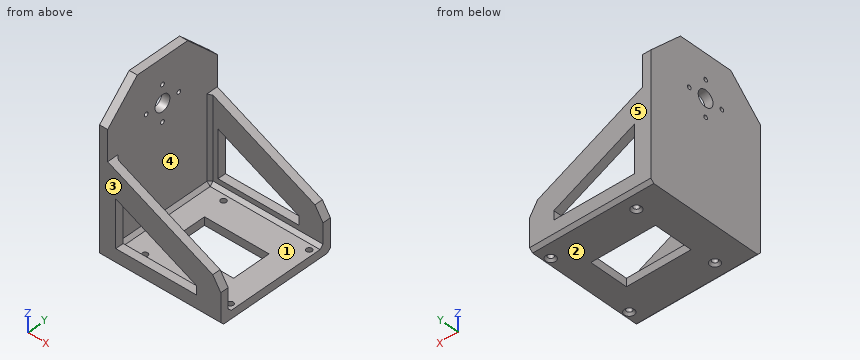
```python
from build123d import *

# Parameters (mm, degrees)
SKETCH004_W      = 75
SKETCH004_H      = 74
SKETCH004_W_2    = 40
SKETCH004_H_2    = 24
PAD_DEPTH        = 5
SKETCH006_W      = 74
SKETCH006_H      = 97
PAD003_DEPTH     = 5
PAD004_DEPTH     = 5
HOLE_D           = 3.4
HOLE_CSINK_D     = 6.1
HOLE_CSINK_ANGLE = 90
SKETCH002_R      = 5
SKETCH002_R_2    = 1.25
POCKET_DEPTH     = 5.001
CHAMFER_SIZE     = 2
CHAMFER001_SIZE  = 5.5
CHAMFER002_SIZE  = 20


with BuildPart() as part:
    # Sketch004 → Pad (new body)
    with BuildSketch(Plane.XY):
        with Locations((32.5, 0)):
            Rectangle(SKETCH004_W, SKETCH004_H)
        with Locations((35, 0)):
            Rectangle(SKETCH004_W_2, SKETCH004_H_2, mode=Mode.SUBTRACT)
    extrude(amount=-PAD_DEPTH)

    # Sketch006 → Pad003 (join)
    with BuildSketch(Plane.YZ):
        with Locations((0, 43.5)):
            Rectangle(SKETCH006_W, SKETCH006_H)
    extrude(amount=-PAD003_DEPTH)

    # Sketch001 → Pad004 (join)
    with BuildSketch(Plane.XZ.offset(37)):
        Polygon((-5, 55.5), (70, 20), (70, -5), (-5, -5), align=None)
        Polygon((5, 34.171185), (55, 10.504519), (55, 5), (5, 5), align=None, mode=Mode.SUBTRACT)
    pad004 = extrude(amount=-PAD004_DEPTH)

    # Mirrored: Pad004 across XZ
    add(pad004.mirror(Plane.XZ))

    # Hole (through all)
    with Locations(Plane(origin=(0, 0, -5), x_dir=(1, 0, 0), z_dir=(0, 0, -1))):
        with Locations((66.5, -26.5), (13.5, -26.5), (13.5, 26.5), (66.5, 26.5)):
            CounterSinkHole(HOLE_D / 2, HOLE_CSINK_D / 2, counter_sink_angle=HOLE_CSINK_ANGLE)

    # Sketch002 → Pocket (cut, through all)
    with BuildSketch(Plane.YZ):
        with Locations((0, 65.5)):
            Circle(SKETCH002_R)
        with Locations((0, 76.5)):
            Circle(SKETCH002_R_2)
        with Locations((11, 65.5)):
            Circle(SKETCH002_R_2)
        with Locations((0, 54.5)):
            Circle(SKETCH002_R_2)
        with Locations((-11, 65.5)):
            Circle(SKETCH002_R_2)
    extrude(amount=-POCKET_DEPTH, mode=Mode.SUBTRACT)

    # Chamfer
    chamfer_edges = [part.edges().sort_by_distance(p)[0] for p in [
        (0, 0, 0),
        (35, 32, 0),
        (35, -32, 0),
        (0, -32, 26.566667),
        (0, 32, 26.566667),
        (32.5, -37, -5),
        (32.5, 37, -5),
    ]]
    chamfer(chamfer_edges, length=CHAMFER_SIZE)

    # Chamfer001
    chamfer001_edges = [part.edges().sort_by_distance(p)[0] for p in [
        (70, -34.5, 20),
        (70, 34.5, 20),
    ]]
    chamfer(chamfer001_edges, length=CHAMFER001_SIZE)

    # Chamfer002
    chamfer002_edges = [part.edges().sort_by_distance(p)[0] for p in [
        (-2.5, -37, 92),
        (-2.5, 37, 92),
    ]]
    chamfer(chamfer002_edges, length=CHAMFER002_SIZE)


solid = part.part
```
Geometry check sheet. Reference: the model listing, model coordinates, mm. Face numbers are marked on the shaded views. A direction names the side the tool comes from. Give positions to 0.01 mm unless a question says otherwise; leave off trailing zeros. Write each loop counter-clockwise with the first axis right and the second up, starting at its lowest first coordinate (ties: lowest second). Pieces come first, ordered by that corner, then holes.
1) Material ranges on L1, parallel to Y at x = 13.5, z = -2.25; L2, parallel to X at y = -26.5, z = -2.7; L3, parallel to X at y = -23, z = 42, recorded low to high.
2) Gauge pin test, flat ends, axial feed: pin 1 (12 mm diameter, centred on y = -8, z = 54, fed in from +X); pin 2 (1.5 mm diameter, centred on y = 34.5, z = 22, fed in from +X); pin 3 (4 mm diameter, centred on x = 36.5, y = -35, fed in from +Z). Record the tip position at first contact, or that the pin passes through.
3) Section check D-D, the plane y = -26.5. Record the boundary of the cut face in (x, z), and give its area (3 significant figures).
4) Section check B-B, the plane y = -7. Record the boundary of the cut face in (x, z).
5) Access from +Z, -Z, +X, -X, +Y, -Y to the whole of each face (thin tool, end or side, straight path). Record for the marked faces 1 and 2.
6) Section check C-C, the plane z = 65.5. Record the boundary of the cut face in (x, y).
7) Section check A-A, the plane z = 6.5. Record the boundary of the cut face in (x, y), and give its area (3 significant figures).
8) Release check for a two-part mould opening along Y. For the marked faces 3, 4 and 5 record: pulls with the +Y half, pulls with the -Y half, needs draft (parallel to the pull), parting line crosses it, or undercut.
Computed:
1. L1: y = -37 to -28.2, -24.8 to 24.8, 28.2 to 37
1. L2: x = -5 to 11.8, 15.2 to 64.8, 68.2 to 70
1. L3: x = -5 to 0
2. pin 1: stops at x = 0
2. pin 2: stops at x = 65.73
2. pin 3: stops at z = 36.8
3. outline: (-5, -5) - (10.45, -5) - (11.8, -3.65) - (11.8, 0) - (2, 0) - (0, 2) - (0, 82.5) - (-5, 82.5) - close; (15.2, -3.65) - (16.55, -5) - (63.45, -5) - (64.8, -3.65) - (64.8, 0) - (15.2, 0) - close; (68.2, -3.65) - (69.55, -5) - (70, -5) - (70, 0) - (68.2, 0) - close
3. area: 752 mm2
4. outline: (-5, -5) - (15, -5) - (15, 0) - (2, 0) - (0, 2) - (0, 92) - (-5, 92) - close; (55, -5) - (70, -5) - (70, 0) - (55, 0) - close
5. face 1: +Z, +X
5. face 2: -Z, +X, -X, +Y, -Y
6. outline: (-5, -37) - (0, -37) - (0, -12.25) - (-5, -12.25) - close; (-5, -9.75) - (0, -9.75) - (0, -5) - (-5, -5) - close; (-5, 5) - (0, 5) - (0, 9.75) - (-5, 9.75) - close; (-5, 12.25) - (0, 12.25) - (0, 37) - (-5, 37) - close
7. outline: (-5, -37) - (5, -37) - (5, -32) - (2, -32) - (0, -30) - (0, 30) - (2, 32) - (5, 32) - (5, 37) - (-5, 37) - close; (55, -37) - (70, -37) - (70, -32) - (55, -32) - close; (55, 32) - (70, 32) - (70, 37) - (55, 37) - close
7. area: 574 mm2
8. face 3: pulls with the -Y half
8. face 4: undercut
8. face 5: pulls with the +Y half
